The model under review builds one solid part; all positions refer to its coordinate system, in mm. Give positions to 0.01 mm unless a question says otherwise; leave off trailing zeros. Loops run counter-clockwise (first coordinate to the right, second up) from the corner with the lowest first, then second, coordinate; pieces in that order, holes last. Notation, with made-up numbers: M 5.5,-30 L 22.5,-30 A9 cw 22.5,-15 Z; hole C 20.25,20 d3. An arc over 180 degrees is marked long. Write item = value, one per line. Start each with the question number.
1. We need section B-B on z = 3. Count the separate pieces of the cut face and the enclosed holes in it, then the cut area to 3 significant figures.
2. We need section A-A on y = 57.15. Give the boundary of the cut face in (x, z) (3 decimals), then the cut area to 3 significant figures.
3. Wall thickness on line 1 along X through (y, z) = (-82, -0.5) (3 decimals); line 2 along X through (y, z) = (16, 5.25) (3 decimals); line 3 along Z through (x, y) = (-72, -90): over which ranges is each line inside the solid? List them lowest first. Write a range as from..to.
4. Draft analysis for pull direction Y (two halves, no side actions). For faces 1 (the face through (-1, 106.362, 0)), 2 (the face through (-71.06, 22.45, 0.86)), 3 (the face through (-1.29, -101.67, 1.52)), 4 (the face through (92.075, -1, 0)), state which applies: pulls with the +Y half, pulls with the -Y half, needs draft (parallel to the pull), parting line crosses it, or undercut.
5. For pin 1 (15.5 mm diameter, centred on x = 76.2, y = -47.625, fed in from +Z); pin 2 (9 mm diameter, centred on x = 76.2, y = 22.225, fed in from +Z); pin 3 (12.5 mm diameter, centred on x = 76.2, y = -12.7, fed in from +Z); pin 4 (11.5 mm diameter, centred on x = -76.2, y = -47.625, fed in from +Z), all flat-tipped, find the tip position at first contact; note any pin that passes through.
from build123d import *

# Parameters (mm, degrees)
SKETCH1_W                                           = 184.15
SKETCH1_H                                           = 212.725
BOSS_EXTRUDE1_DEPTH                                 = 6.35
CSK_FOR_3_8_FLAT_HEAD_SOCKET_CAP_SCREW1_D           = 9.8044
CSK_FOR_3_8_FLAT_HEAD_SOCKET_CAP_SCREW1_CSINK_D     = 19.8374
CSK_FOR_3_8_FLAT_HEAD_SOCKET_CAP_SCREW1_CSINK_ANGLE = 82
CHAMFER1_SIZE                                       = 9.525


with BuildPart() as part:
    # Sketch1 → Boss-Extrude1 (new body, symmetric)
    with BuildSketch(Plane.XY):
        Rectangle(SKETCH1_W, SKETCH1_H)
    extrude(amount=BOSS_EXTRUDE1_DEPTH, both=True)

    # CSK for 3/8 Flat Head Socket Cap Screw1 (through all)
    with Locations(Plane.XY.offset(6.35)):
        with Locations((-76.2, 92.075), (-76.2, 57.15), (-76.2, 22.225), (-76.2, -12.7), (-76.2, -47.625), (-76.2, -82.55), (76.2, -82.55), (76.2, -47.625), (76.2, -12.7), (76.2, 22.225), (76.2, 57.15), (76.2, 92.075)):
            CounterSinkHole(CSK_FOR_3_8_FLAT_HEAD_SOCKET_CAP_SCREW1_D / 2, CSK_FOR_3_8_FLAT_HEAD_SOCKET_CAP_SCREW1_CSINK_D / 2, counter_sink_angle=CSK_FOR_3_8_FLAT_HEAD_SOCKET_CAP_SCREW1_CSINK_ANGLE)

    # Chamfer1
    chamfer1_edges = [part.edges().sort_by_distance(p)[0] for p in [
        (0, -106.3625, 6.35),
    ]]
    chamfer(chamfer1_edges, length=CHAMFER1_SIZE)


solid = part.part
Final values:
q1.separate_pieces = 1
q1.enclosed_holes = 12
q1.area = 36,200 mm²
q2.outline = M -92.075,-6.35 L -81.102,-6.35 L -81.102,0.579 L -86.119,6.35 L -92.075,6.35 Z; M -71.298,-6.35 L 71.298,-6.35 L 71.298,0.579 L 66.281,6.35 L -66.281,6.35 L -71.298,0.579 Z; M 81.102,-6.35 L 92.075,-6.35 L 92.075,6.35 L 86.119,6.35 L 81.102,0.579 Z
q2.area = 2,030 mm²
q3.line_1 = -92.075..-81.071, -71.329..71.329, 81.071..92.075
q3.line_2 = -92.075..-82.648, -69.752..69.752, 82.648..92.075
q3.line_3 = -6.35..4.78
q4.face_1 = pulls with the +Y half
q4.face_2 = undercut
q4.face_3 = pulls with the -Y half
q4.face_4 = needs draft
q5.pin_1 = 3.86
q5.pin_2 = through
q5.pin_3 = 2.13
q5.pin_4 = 1.55
